Part model, mm, in its own coordinate system. A direction names the side the tool comes from. Round coordinates to 2 decimals unless told otherwise and drop trailing zeros. Order: outer loops, then holes, each group sorted by start corner. A loop starts at its lowest first (then second) coordinate and runs counter-clockwise, first axis right, second up. Notation, with made-up numbers: (52.25, 42) - (61.25, 42) arc R30 ccw to (61.25, 65) - close; hole circle Ø8 at (-33.75, 30). An arc over 180 degrees is marked (long way). Answer as a JSON object with one key per item and string values.
Autodesk Inventor part; units mm, degrees
ref_plane "YZ Plane" through (0, 0, 0) normal (1, 0, 0) x (0, 1, 0)
ref_plane "XZ Plane" through (0, 0, 0) normal (0, 1, 0) x (-1, 0, 0)
ref_plane "XY Plane" through (0, 0, 0) normal (0, 0, 1) x (1, 0, 0)
sketch "スケッチ1" plane through (0, 0, 0) normal (0, 0, 1) x (1, 0, 0)
  line L0 (-28, -31.5) -> (28, -31.5) construction
  line L1 (28, -31.5) -> (28, 31.5) construction
  line L2 (28, 31.5) -> (-28, 31.5) construction
  line L3 (-28, 31.5) -> (-28, -31.5) construction
  line L4 (-28, -31.5) -> (28, 31.5) construction
  line L5 (28, -31.5) -> (-28, 31.5) construction
  line L6 (-28, 10.6) -> (-28, 31.5)
  line L7 (-28, 31.5) -> (28, 31.5)
  line L8 (28, 31.5) -> (28, 10.6)
  line L9 (-28, -10.6) -> (-28, -31.5)
  line L10 (-28, -31.5) -> (28, -31.5)
  line L11 (28, -31.5) -> (28, -10.6)
  line L12 (-28, 8.5) -> (-33, 8.5)
  line L13 (-33, 8.5) -> (-33, -8.5)
  line L14 (-33, -8.5) -> (-28, -8.5)
  line L15 (28, 8.5) -> (33, 8.5)
  line L16 (33, 8.5) -> (33, -8.5)
  line L17 (33, -8.5) -> (28, -8.5)
  line L18 (0, 0) -> (0, 31.5) construction
  line L19 (0, 0) -> (28, 0) construction
  arc A0 (-28, 8.5) -> (-28, 10.6) centre (-28, 9.55) ccw
  arc A1 (-28, -10.6) -> (-28, -8.5) centre (-28, -9.55) ccw
  arc A2 (28, 10.6) -> (28, 8.5) centre (28, 9.55) ccw
  arc A3 (28, -8.5) -> (28, -10.6) centre (28, -9.55) ccw
  dimension "d45" = 63
  dimension "d73" = 56
  dimension "d74" = 1.05
  dimension "d75" = 5
  dimension "d76" = 23
extrude "押し出し1" add sketch "スケッチ1" along normal blind 5
sketch "スケッチ2" plane through (0, 0, 5) normal (0, 0, 1) x (1, 0, 0)
  line L0 (-28, 31.5) -> (-28, 10.6)
  line L1 (28, 10.6) -> (28, 31.5)
  line L2 (-50.9845, 57.5344) -> (-28, 57.5344)
  line L3 (-28, 57.5344) -> (-28, -57.37)
  line L4 (-28, -57.37) -> (-50.9845, -57.37)
  line L5 (-50.9845, -57.37) -> (-50.9845, 57.5344)
  line L6 (28, 64.7229) -> (65.0267, 64.7229)
  line L7 (65.0267, 64.7229) -> (65.0267, -57.37)
  line L8 (65.0267, -57.37) -> (28, -57.37)
  line L9 (28, -57.37) -> (28, 64.7229)
  point P0 (0, 0)
extrude "押し出し2" cut sketch "スケッチ2" against normal blind 2.5
sketch "スケッチ3" plane through (28, -31.5, 0) normal (1, 0, 0) x (0, 0, -1)
  line L0 (0, 0) -> (-5, 0)
  line L1 (0, 63) -> (-5, 63)
  point P0 (0, 31.5)
  point P1 (-2.5, 8)
  point P2 (-2.5, 55)
  point P3 (-2.5, 0)
  dimension "d81" = 8
  dimension "d82" = 8
hole "穴1" at (28, -23.5, 2.5) at (28, 23.5, 2.5) direction (-1, 0, 0) diameter 2.459 depth 2.5
mirror "ミラー1" about plane through (0, 0, 0) normal (1, 0, 0) of "穴1"
sketch "スケッチ4" plane through (0, 0, 5) normal (0, 0, 1) x (1, 0, 0)
  line L0 (-28, -31.5) -> (28, -31.5)
  line L1 (28, -31.5) -> (28, -10.6)
  line L2 (18, 26.5) -> (-18, 26.5)
  line L3 (-18, 26.5) -> (-18, -26.5)
  line L4 (-18, -26.5) -> (18, -26.5)
  line L5 (18, -26.5) -> (18, 26.5)
  line L6 (18, 26.5) -> (-18, -26.5) construction
  line L7 (-18, 26.5) -> (18, -26.5) construction
  point P0 (0, 0)
  dimension "d90" = 10
  dimension "d91" = 5
extrude "押し出し3" cut sketch "スケッチ4" against normal blind 10
fillet "フィレット1" radius 10 4 edges at (18, -26.5, 2.5) (-18, -26.5, 2.5) (-18, 26.5, 2.5) (18, 26.5, 2.5)
equation "\"d45\" = d1"
equation "\"d76\" = d20 + d23"
properties part number "コックピット_2_サブフレーム_4" material "アセタール樹脂、黒"
Item 1: Cut at C-C (y = 13.5). Write the cut outline in (x, z).
Taken from the geometry:
{"outline": "(-28, 0) - (-18, 0) - (-18, 5) - (-28, 5) - close; (18, 0) - (28, 0) - (28, 5) - (18, 5) - close"}
Item 2: Two-plate mould, pull along Y, no slides. Class faces 1 (the flat face through (-31, -8.5, 1)), 2 (the cylindrical face through (-14.99, -23.65, 2.46)), 3 (the flat face through (-28, 0, 4)), 4 (the flat face through (0, 31.5, 2)): pulls with the +Y half, pulls with the -Y half, needs draft (parallel to the pull), parting line crosses it, or undercut.
Taken from the geometry:
{"face 1": "pulls with the -Y half", "face 2": "undercut", "face 3": "needs draft", "face 4": "pulls with the +Y half"}
Item 3: Cut at D-D (x = 29). Write the cut outline in (y, z), plus the area to 3 significant figures.
Taken from the geometry:
{"outline": "(-8.5, 0) - (8.5, 0) - (8.5, 2.5) - (-8.5, 2.5) - close", "area": "42.5 mm2"}
Item 4: Drop flat-ended pins along their axis: P1, Ø1.5, axis at y = -23.5, z = 1.5, coming from the +X side; P2, Ø2.5, axis at y = 18, z = 3.5, coming from the -X side; P3, Ø2, axis at x = 29.5, z = 1, coming from the -Y side. Give the stop position or say it passes through.
Taken from the geometry:
{"P1": "x = 28", "P2": "x = -28", "P3": "y = -8.5"}
Item 5: Cut at B-B (x = -5.5). Write the cut outline in (y, z), plus the area to 3 significant figures.
Taken from the geometry:
{"outline": "(-31.5, 0) - (-26.5, 0) - (-26.5, 5) - (-31.5, 5) - close; (26.5, 0) - (31.5, 0) - (31.5, 5) - (26.5, 5) - close", "area": "50.0 mm2"}
Item 6: Cut at A-A (y = 6). Write the cut outline in (x, z), plus the area to 3 significant figures.
Taken from the geometry:
{"outline": "(-33, 0) - (-18, 0) - (-18, 5) - (-28, 5) - (-28, 2.5) - (-33, 2.5) - close; (18, 0) - (33, 0) - (33, 2.5) - (28, 2.5) - (28, 5) - (18, 5) - close", "area": "125 mm2"}
Item 7: Tool access for faces 5 (the flat face through (25.5, -24, 3)), 6 (the cylindrical face through (-15.15, 23.49, 2.46)), 7 (the flat face through (-31, 0, 2.5)), 8 (the flat face through (28, 21, 2)): list every direction of +Z, -Z, +X, -X, +Y, -Y with a clear straight run to the whole face (end or side of a thin tool).
Taken from the geometry:
{"face 5": "+X", "face 6": "+Z, -Z", "face 7": "+Z, -X, +Y, -Y", "face 8": "+Z, -Z, +X, +Y"}
Item 8: Probe L1, parallel to Y at x = 26.85, z = 2.5; L2, parallel to Y at x = -5.5, z = 2.4; L3, parallel to Z at x = -27.35, y = 23.5. List the from-to ranges inside material, lowest first. Write a range as from..to.
Taken from the geometry:
{"L1": "-31.5..-24.73, -22.27..22.27, 24.73..31.5", "L2": "-31.5..-26.5, 26.5..31.5", "L3": "0..1.27, 3.73..5"}
